Could you check a few things on this model? Use its own coordinates, in mm. A direction names the side the tool comes from. Give positions to 0.01 mm unless a question says otherwise; leave off trailing zeros. Loops run counter-clockwise (first coordinate to the right, second up) from the corner with the lowest first, then second, coordinate; pieces in that order, holes last. Notation, with made-up numbers: (-2, 82.5) - (6, 82.5) arc R20 cw to (6, 106.5) - close; hole circle Ø11 at (-34.5, 46). An arc over 180 degrees is marked (long way). Use CSV: the item, a comma, the result in double quotes.
from build123d import *

# Parameters (mm, degrees)
SKETCH006_W   = 13
SKETCH006_H   = 2.5
PAD006_DEPTH  = 3
SKETCH005_R   = 3
SKETCH005_W   = 15
SKETCH005_H   = 6
SKETCH005_W_2 = 9
SKETCH005_H_2 = 3
PAD005_DEPTH  = 3
SKETCH004_W   = 16
SKETCH004_H   = 14
SKETCH004_H_2 = 17
PAD004_DEPTH  = 3
SKETCH003_W   = 92
SKETCH003_H   = 63
SKETCH003_W_2 = 88
SKETCH003_H_2 = 59
PAD003_DEPTH  = 24
SKETCH002_W   = 88
SKETCH002_H   = 59
PAD002_DEPTH  = 2
SKETCH_R      = 1.1
PAD_DEPTH     = 6.5
SKETCH001_R   = 3
PAD001_DEPTH  = 5


with BuildPart() as pad006:
    # Sketch006 → Pad006 (new body)
    with BuildSketch(Plane.YZ.offset(88)):
        with Locations((-27.5, 3.75)):
            Rectangle(SKETCH006_W, SKETCH006_H)
    extrude(amount=PAD006_DEPTH)


with BuildPart() as pad005:
    # Sketch005 → Pad005 (new body)
    with BuildSketch(Plane(origin=(0, 0, 0), x_dir=(-1, 0, 0), z_dir=(0, 1, 0))):
        with Locations((-31.5, 9)):
            Circle(SKETCH005_R)
        with Locations((-53, 9)):
            Rectangle(SKETCH005_W, SKETCH005_H)
        with Locations((-74.4, 7.5)):
            Rectangle(SKETCH005_W_2, SKETCH005_H_2)
    extrude(amount=PAD005_DEPTH)


with BuildPart() as pad004:
    # Sketch004 → Pad004 (new body)
    with BuildSketch(Plane(origin=(0, 0, 0), x_dir=(0, -1, 0), z_dir=(-1, 0, 0))):
        with Locations((11, 13)):
            Rectangle(SKETCH004_W, SKETCH004_H)
        with Locations((30, 14.5)):
            Rectangle(SKETCH004_W, SKETCH004_H_2)
        with Locations((48, 14.5)):
            Rectangle(SKETCH004_W, SKETCH004_H_2)
    extrude(amount=PAD004_DEPTH)


with BuildPart() as cut003:
    # Sketch003 → Pad003 (new body)
    with BuildSketch(Plane.XY):
        with Locations((44, -29.5)):
            Rectangle(SKETCH003_W, SKETCH003_H)
        with Locations((44, -29.5)):
            Rectangle(SKETCH003_W_2, SKETCH003_H_2, mode=Mode.SUBTRACT)
    extrude(amount=PAD003_DEPTH)

    # Cut001: cut Pad004
    add(pad004.part, mode=Mode.SUBTRACT)

    # Cut002: cut Pad005
    add(pad005.part, mode=Mode.SUBTRACT)

    # Cut003: cut Pad006
    add(pad006.part, mode=Mode.SUBTRACT)


with BuildPart() as base:
    # Sketch002 → Pad002 (new body)
    with BuildSketch(Plane.XY):
        with Locations((44, -29.5)):
            Rectangle(SKETCH002_W, SKETCH002_H)
    extrude(amount=PAD002_DEPTH)


with BuildPart() as pad:
    # Sketch → Pad (new body)
    with BuildSketch(Plane.XY.offset(2.5)):
        with Locations((23.5, -3.5)):
            Circle(SKETCH_R)
        with Locations((23.5, -52.5)):
            Circle(SKETCH_R)
        with Locations((81.5, -3.5)):
            Circle(SKETCH_R)
        with Locations((81.5, -52.5)):
            Circle(SKETCH_R)
    extrude(amount=PAD_DEPTH)


with BuildPart() as fusion001:
    # Sketch001 → Pad001 (new body)
    with BuildSketch(Plane.XY.offset(4)):
        with Locations((23.5, -3.5)):
            Circle(SKETCH001_R)
        with Locations((81.5, -3.5)):
            Circle(SKETCH001_R)
        with Locations((81.5, -52.5)):
            Circle(SKETCH001_R)
        with Locations((23.5, -52.5)):
            Circle(SKETCH001_R)
    extrude(amount=PAD001_DEPTH)

    # Cut: cut Pad
    add(pad.part, mode=Mode.SUBTRACT)


with BuildPart() as fusion001_1:
    # Cut placement: moved
    add(fusion001.part.moved(Location((0.000478, -1.138495, -3.808742))))

    # Fusion: union Base
    add(base.part)

    # Fusion001: union Cut003
    add(cut003.part)


solid = fusion001_1.part
1) I'm going to push flat-ended pins straight in: P1, Ø3, axis at x = 23.5, y = -4.64, coming from the +Z side; P2, Ø0.7, axis at x = 23.5, y = -53, coming from the +Z side. Where does each tip first touch, or does it pass through?
Answer below:
P1,"stops at z = 5.19"
P2,"stops at z = 2"
2) Suppose I cut it at A-A (z = 16.5). Please give me the cut outline in (x, y), plus the area to 3 significant figures.
Answer below:
outline,"(-2, -61) - (90, -61) - (90, 2) - (-2, 2) - (-2, -3) - (0, -3) - (0, 0) - (88, 0) - (88, -59) - (0, -59) - (0, -56) - (-2, -56) - close; (-2, -40) - (0, -40) - (0, -38) - (-2, -38) - close; (-2, -22) - (0, -22) - (0, -19) - (-2, -19) - close"
area,"508 mm2"
3) Suppose I cut it at D-D (y = -28). Please give me the cut outline in (x, z).
Answer below:
outline,"(-2, 0) - (90, 0) - (90, 2.5) - (88, 2.5) - (88, 2) - (0, 2) - (0, 6) - (-2, 6) - close; (-2, 23) - (0, 23) - (0, 24) - (-2, 24) - close; (88, 5) - (90, 5) - (90, 24) - (88, 24) - close"
4) Suppose I cut it at C-C (x = 31.5). Please give me the cut outline in (y, z).
Answer below:
outline,"(-61, 0) - (2, 0) - (2, 6) - (0, 6) - (0, 2) - (-59, 2) - (-59, 24) - (-61, 24) - close; (0, 12) - (2, 12) - (2, 24) - (0, 24) - close"
5) Which directions (+Z, -Z, +X, -X, +Y, -Y) give clear straight access to the entire face, cutting with the end or side of a thin tool? Please do faces 4 (the flat face through (-1, -30, 23)), 5 (the flat face through (89, -28, 5)), 6 (the flat face through (53, 1, 6)), 7 (the flat face through (23, -54, 2)).
Answer below:
face 4,"-X"
face 5,"+X"
face 6,"+Y"
face 7,"+Z"
6) I need wall thicknesses on line 1 along Y through (x, z) = (14, 20); line 2 along X through (y, z) = (-20, 14); line 3 along Z through (x, y) = (31.5, 0.5). Which ranges of each line are inside material? Lowest first, please.
Answer below:
line 1,"y = -61 to -59, 0 to 2"
line 2,"x = -2 to 0, 88 to 90"
line 3,"z = 0 to 6, 12 to 24"
7) We'd pull the mould along X, two halves only. Please class faces 1 (the flat face through (-1, -56, 14)), 2 (the cylindrical face through (80.4, -4.6, 3.6)), 3 (the flat face through (-2, -30, 4)): +X half, -X half, draft (parallel to the pull), parting line (faces both ways), or undercut.
Answer below:
face 1,"draft"
face 2,"undercut"
face 3,"-X half"
8) Suppose I cut it at B-B (y = -35.5). Please give me the cut outline in (x, z), plus the area to 3 significant figures.
Answer below:
outline,"(-2, 0) - (90, 0) - (90, 24) - (88, 24) - (88, 2) - (0, 2) - (0, 6) - (-2, 6) - close; (-2, 23) - (0, 23) - (0, 24) - (-2, 24) - close"
area,"238 mm2"
